Verification items for the finished model (mm, model axes). Face numbers are marked on the shaded views. A direction names the side the tool comes from. Coordinates: 2 decimals unless noted, no trailing zeros. Write each loop counter-clockwise with the first axis right and the second up, starting at its lowest first coordinate (ties: lowest second). Pieces come first, ordered by that corner, then holes. Notation, with made-up numbers: (38, 51) -> (52, 51) arc R24 ccw to (52, 85) -> close; hole circle Ø8 at (82.25, 31). An arc over 180 degrees is marked (long way). Answer in a Markdown table with one row per item.
```python
from build123d import *

# Parameters (mm, degrees)
F0_W         = 7.62
F0_H         = 3.81
F1_DEPTH     = 17.78
F2_W         = 51.562
F2_H         = 1.143
F2_W_2       = 26.162
F3_DEPTH     = 7.62
F4_T4_DEPTH  = 17.78
F4_T9_DEPTH  = 17.78
F4_T14_DEPTH = 17.78
F4_T19_DEPTH = 17.78
F5_R         = 1.5875
F6_DEPTH     = 25.4
F7_R         = 2.0955
F8_DEPTH     = 7.62
F9_R         = 1.27


# Not quite as in the source:
# - a fillet or chamfer that OpenCascade refuses, or shapes differently, is made with other operations: its cross-section is extruded or revolved along the edge and cut away or added


with BuildPart() as f1:
    # F0 (on Top) → F1 (new body)
    with BuildSketch(Plane.XY):
        Polygon((0, 3.683), (0, 0), (12.7, 0), (43.434, 0), (56.134, 0), (56.134, 3.683), align=None)
        Polygon((43.434, 0), (12.7, 0), (12.7, -3.683), (24.257, -3.683), (31.877, -3.683), (43.434, -3.683), align=None)
        with Locations((28.067, -5.588)):
            Rectangle(F0_W, F0_H)
    extrude(amount=F1_DEPTH)

    # F2 (on face) → F3 (cut)
    with BuildSketch(Plane(origin=(0, 0, 0), x_dir=(1, 0, 0), z_dir=(0, 0, -1))):
        with Locations((28.067, -1.8415)):
            Rectangle(F2_W, F2_H)
        with Locations((28.067, 1.8415)):
            Rectangle(F2_W_2, F2_H)
    extrude(amount=-F3_DEPTH, mode=Mode.SUBTRACT)

    # F4: chamfer of 3.81 on 4 edges, made by hand


with BuildPart() as f4_tool2:
    # F4_s3 → F4_t4 (new body)
    with BuildSketch(Plane.XY):
        Polygon((35.687, -3.683), (31.877, -7.493), (31.877, -3.683), align=None)
    extrude(amount=F4_T4_DEPTH)

    split(bisect_by=Plane.XZ.offset(7.493), keep=Keep.BOTTOM)


with BuildPart() as f1_1:
    add(f1.part)

    # F4_t1: union F4_tool2
    add(f4_tool2.part)


with BuildPart() as f4_tool7:
    # F4_s8 → F4_t9 (new body)
    with BuildSketch(Plane.XY):
        Polygon((47.244, 0), (43.434, -3.81), (43.434, 0), align=None)
    extrude(amount=F4_T9_DEPTH)

    split(bisect_by=Plane.XZ.offset(3.683), keep=Keep.BOTTOM)


with BuildPart() as f1_2:
    add(f1_1.part)

    # F4_t6: union F4_tool7
    add(f4_tool7.part)


with BuildPart() as f4_tool12:
    # F4_s13 → F4_t14 (new body)
    with BuildSketch(Plane.XY):
        Polygon((20.447, -3.683), (24.257, -7.493), (24.257, -3.683), align=None)
    extrude(amount=F4_T14_DEPTH)

    split(bisect_by=Plane.XZ.offset(7.493), keep=Keep.BOTTOM)


with BuildPart() as f1_3:
    add(f1_2.part)

    # F4_t11: union F4_tool12
    add(f4_tool12.part)


with BuildPart() as f4_tool17:
    # F4_s18 → F4_t19 (new body)
    with BuildSketch(Plane.XY):
        Polygon((8.89, 0), (12.7, -3.81), (12.7, 0), align=None)
    extrude(amount=F4_T19_DEPTH)

    split(bisect_by=Plane.XZ.offset(3.683), keep=Keep.BOTTOM)


with BuildPart() as f1_4:
    add(f1_3.part)

    # F4_t16: union F4_tool17
    add(f4_tool17.part)

    # F5 (on face) → F6 (cut)
    with BuildSketch(Plane.XZ.offset(7.493)):
        with Locations((28.067, 13.462)):
            Circle(F5_R)
        with Locations((28.067, 4.318)):
            Circle(F5_R)
    extrude(amount=-F6_DEPTH, mode=Mode.SUBTRACT)

    # F7 (on face) → F8 (cut)
    with BuildSketch(Plane.XY.offset(17.78)):
        with Locations((28.067, 0)):
            Circle(F7_R)
    extrude(amount=-F8_DEPTH, mode=Mode.SUBTRACT)

    # F9
    f9_edges = [f1_4.edges().sort_by_distance(p)[0] for p in [
        (0, 0, 8.89),
        (56.134, 0, 8.89),
        (56.134, 3.683, 8.89),
        (0, 3.683, 8.89),
        (12.573, -3.683, 8.89),
        (43.561, -3.683, 8.89),
        (31.877, -7.493, 8.89),
        (24.257, -7.493, 8.89),
        (8.89, 0, 8.89),
        (47.244, 0, 8.89),
        (35.687, -3.683, 8.89),
        (20.447, -3.683, 8.89),
    ]]
    fillet(f9_edges, radius=F9_R)


solid = f1_4.part
```
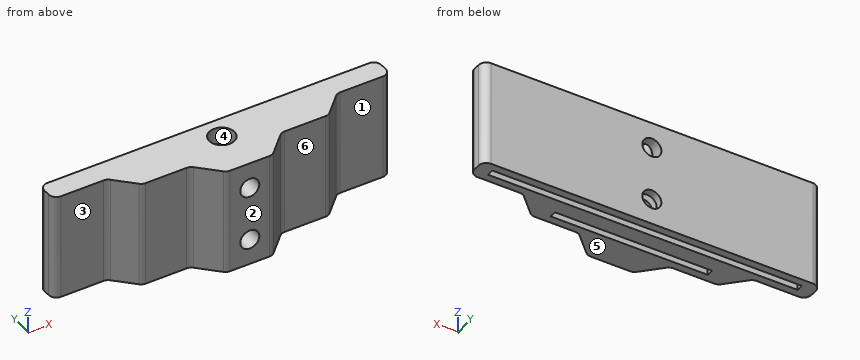
1. Sectioned sample at B-B, the plane x = 5.5. Record the cut outline in (y, z), and give its area (3 significant figures).
Findings below:
| item | result |
|---|---|
| outline | (0, 0) -> (1.27, 0) -> (1.27, 7.62) -> (2.41, 7.62) -> (2.41, 0) -> (3.68, 0) -> (3.68, 17.78) -> (0, 17.78) -> close |
| area | 56.8 mm² |
2. Sectioned sample at A-A, the plane z = 2. Count the separate pieces of the cut face and the enclosed holes in it, and give its area (3 significant figures).
Findings below:
| item | result |
|---|---|
| separate pieces | 1 |
| enclosed holes | 2 |
| area | 288 mm² |
3. Release check for a two-part mould opening along Y. For the marked faces 4, 5 and 6 record: released by +Y, released by -Y, zero draft, split by the parting line, or undercut.
Findings below:
| item | result |
|---|---|
| face 4 | undercut |
| face 5 | zero draft |
| face 6 | released by -Y |
4. Access from +Z, -Z, +X, -X, +Y, -Y to the whole of each face (thin tool, end or side, straight path). Record for the marked faces 1, 2 and 3.
Findings below:
| item | result |
|---|---|
| face 1 | +Z, -Z, +X, -Y |
| face 2 | +Z, -Z, +X, -X, -Y |
| face 3 | +Z, -Z, -X, -Y |
5. Sectioned sample at D-D, the plane y = -5. Record the cut outline in (x, z) (1 decimal).
Findings below:
| item | result |
|---|---|
| outline | (21.8, 0) -> (34.4, 0) -> (34.4, 17.8) -> (21.8, 17.8) -> close; hole circle Ø3.2 at (28.1, 4.3); hole circle Ø3.2 at (28.1, 13.5) |
6. Material ranges on probe 1 along Y at (x, z) = (30.5, 4.5); probe 2 along Y at (x, z) = (4.5, 1.5); probe 3 along Z at (x, y) = (29, -3.75), recorded low to high. Write a range as from..to.
Findings below:
| item | result |
|---|---|
| probe 1 | y = -7.49..-2.41, -1.27..1.27, 2.41..3.68 |
| probe 2 | y = 0..1.27, 2.41..3.68 |
| probe 3 | z = 0..3.03, 5.6..12.18, 14.75..17.78 |
7. Go/stop test with flat-tipped pins: pin 1 (3.5 mm diameter, centred on x = 5, z = 10.5, fed in from -Y); pin 2 (8 mm diameter, centred on x = 44.5, z = 15.5, fed in from -Y); pin 3 (3 mm diameter, centred on x = 28.067, z = 13.462, fed in from -Y); pin 4 (0.6 mm diameter, centred on y = -2, z = 3, fed in from +X). Record where each tip stops, or that it passes through.
Findings below:
| item | result |
|---|---|
| pin 1 | stops at y = 0 |
| pin 2 | stops at y = -3.68 |
| pin 3 | passes through |
| pin 4 | stops at x = 45.54 |
